The listing builds one solid part. Answer for the finished solid, in the listing's coordinates (mm). Give positions to 0.01 mm unless a question says otherwise; leave off trailing zeros. Loops run counter-clockwise (first coordinate to the right, second up) from the corner with the lowest first, then second, coordinate; pieces in that order, holes last. Notation, with made-up numbers: (76.25, 7) - (118.25, 7) arc R10 ccw to (118.25, 17) - close; hole circle Ø4 at (17.5, 22). An arc over 180 degrees is marked (long way). Write each question's results on one line, items separated by ' | '.
from build123d import *

# Parameters (mm, degrees)
BOSS_EXTRUDE1_DEPTH      = 76.2
F_8_0_8_DIAMETER_HOLE1_D = 8


with BuildPart() as part:
    # Sketch1 → Boss-Extrude1 (new body)
    with BuildSketch(Plane.XY):
        with BuildLine():
            Line((3.859161178, -5.75), (-3.859161178, -5.75))
            ThreePointArc((-3.859161178, -5.75), (-6.925, 0), (-3.859161178, 5.75))
            Line((-3.859161178, 5.75), (3.859161178, 5.75))
            ThreePointArc((3.859161178, 5.75), (6.925, 0), (3.859161178, -5.75))
        make_face()
    extrude(amount=BOSS_EXTRUDE1_DEPTH)

    # 8.0 _8_ Diameter Hole1 (through all)
    with Locations(Plane(origin=(0, 0, 0), x_dir=(-1, 0, 0), z_dir=(0, 0, -1))):
        with Locations((0, 0)):
            Hole(F_8_0_8_DIAMETER_HOLE1_D / 2)


solid = part.part
Item 1: A cutting plane is placed at B-B, the plane y = 0. Determine the outline of the cut face in (x, z) (3 decimals).
Values found:
outline: (-6.925, 0) - (-4, 0) - (-4, 76.2) - (-6.925, 76.2) - close; (4, 0) - (6.925, 0) - (6.925, 76.2) - (4, 76.2) - close
Item 2: A cutting plane is placed at D-D, the plane x = 6.25. Determine the outline of the cut face in (y, z).
Values found:
outline: (-2.98, 0) - (2.98, 0) - (2.98, 76.2) - (-2.98, 76.2) - close
Item 3: Find the intervals of material crossed by line 1 along Y through (x, z) = (0, 37); line 2 along X through (y, z) = (-1.5, 67.5); line 3 along Y through (x, z) = (2.25, 72), in increasing order. Write a range as [from, to].
Values found:
line 1: y = [-5.75, -4], [4, 5.75] | line 2: x = [-6.76, -3.71], [3.71, 6.76] | line 3: y = [-5.75, -3.31], [3.31, 5.75]
Item 4: Flat-ended cylindrical pins translate along their axes: P1, Ø5, axis at y = 3.5, z = 43, coming from the -X side; P2, Ø1.5, axis at x = 2.5, y = -1, coming from the +Z side; P3, Ø1, axis at y = -3, z = 56.5, coming from the +X side; P4, Ø4, axis at y = -3, z = 17.5, coming from the +X side. Find the tip coordinate at first contact, or state that the pin passes through.
Values found:
P1: stops at x = -6.85 | P2: passes through | P3: stops at x = 6.46 | P4: stops at x = 6.85
Item 5: A cutting plane is placed at C-C, the plane z = 64. Determine the outline of the cut face in (x, y) (3 decimals), plus the area to 3 significant figures.
Values found:
outline: (-3.859, -5.75) - (3.859, -5.75) arc R6.925 ccw to (3.859, 5.75) - (-3.859, 5.75) arc R6.925 ccw to start; hole circle Ø8 at (0, 0) | area: 88.1 mm²
Item 6: For a pull along X with two mould halves and no side action, classify faces 1 (the face through (2, -4, 0)), 2 (the face through (6.924, 0.095, 37.567)), 3 (the face through (-0.867, -3.905, 38.633)), 4 (the face through (-6.924, -0.095, 37.567)) as released by +X, released by -X, zero draft, split by the parting line, or undercut.
Values found:
face 1: zero draft | face 2: released by +X | face 3: undercut | face 4: released by -X
Item 7: A cutting plane is placed at A-A, the plane x = 0. Determine the outline of the cut face in (y, z).
Values found:
outline: (-5.75, 0) - (-4, 0) - (-4, 76.2) - (-5.75, 76.2) - close; (4, 0) - (5.75, 0) - (5.75, 76.2) - (4, 76.2) - close
